Geometry check sheet. Reference: drawing and pictorial views, mm from the part's lowest x, y, z. Give positions to 0.01 mm unless a question says otherwise; leave off trailing zeros. Order: outer loops, then holes, each group sorted by start corner. A loop starts at its lowest first (then second) coordinate and runs counter-clockwise, first axis right, second up. Notation, with made-up numbers: M 21,60.25 L 74,60.25 A25 ccw 74,78.25 Z; hole C 70.5,34.5 d6. An arc over 180 degrees is marked long. Answer as CSV lines item,"result".
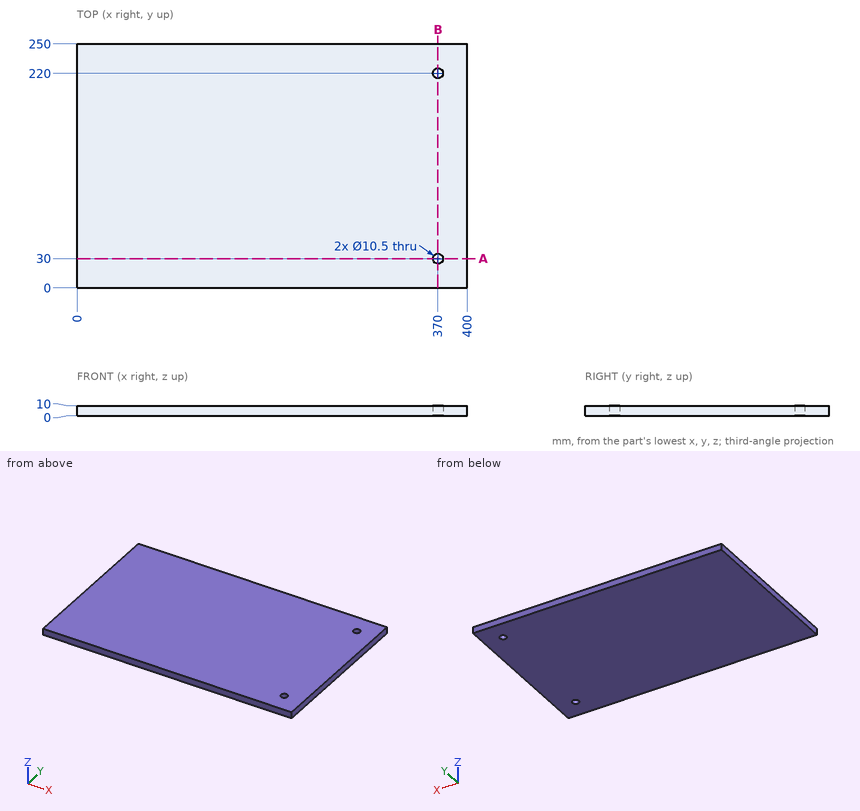
(1) Section check B-B on x = 370. Enter the section's corners in (y, z).
The answers:
outline,"M 0,0 L 24.75,0 L 24.75,10 L 0,10 Z; M 35.25,0 L 214.75,0 L 214.75,10 L 35.25,10 Z; M 225.25,0 L 250,0 L 250,10 L 225.25,10 Z"
(2) Section check A-A on y = 30. Enter the section's corners in (x, z), then the cut area to 4 significant figures.
The answers:
outline,"M 0,0 L 364.75,0 L 364.75,10 L 0,10 Z; M 375.25,0 L 400,0 L 400,10 L 375.25,10 Z"
area,"3,895 mm2"
(3) Material ranges on line 1 (Y direction, x = 370, z = 3.5), recorded low to high.
The answers:
line 1,"y = 0 to 24.75, 35.25 to 214.75, 225.25 to 250"
(4) Gauge pin test, flat end, axial feed: P1, Ø12, axis at x = 370, y = 30, coming from the +Z side. Record the tip position at first contact, or that the pin passes through.
The answers:
P1,"stops at z = 10"
